Design review of the part built by this model. Coordinates are the model's own, in mm. A direction names the side the tool comes from. Coordinates: 2 decimals unless noted, no trailing zeros. Write each loop counter-clockwise with the first axis right and the second up, starting at its lowest first coordinate (ties: lowest second). Pieces come first, ordered by that corner, then holes. Notation, with made-up numbers: (22, 67.25) -> (34, 67.25) arc R23 ccw to (34, 82.25) -> close; hole circle Ø11 at (24, -15). An arc over 180 degrees is marked (long way). One line per question, with ' | ' between items. Start each with the question number.
Q1. Wall thickness on probe 1 along Z at (x, y) = (57.15, 2.25); probe 2 along X at (y, z) = (4.5, -6.55) (3 decimals); probe 3 along X at (y, z) = (5, 25.4) (3 decimals): over which ranges is each line inside the solid? List them lowest first.
Q2. For faces 1 (the flat face through (27, 3, 0)), 2 (the cylindrical face through (55.563, 3.131, 26.617)), list the 3-axis set-ups (+Z, -Z, +X, -X, +Y, -Y) from which the entire face can be reached by the end or side of a thin tool; tool diameter is ignored.
Q3. Add section C-C on z = -19.05. State the section outline as (x, y) points (3 decimals), and give its area (3 significant figures).
Q4. Add section D-D on y = 3. State the section outline as (x, z) points (3 decimals).
Q5. For P1, Ø1.9, axis at x = 37, y = 3, coming from the +Z side, flat-tipped, find the tip position at first contact; note if it passes through.
Q6. Add section A-A on z = -6.55. State the section outline as (x, y) points (3 decimals), and give its area (3 significant figures).
Q7. Add section B-B on x = 57.15. State the section outline as (y, z) points.
from build123d import *

# Parameters (mm, degrees)
SKETCH1_R           = 2
BOSS_EXTRUDE1_DEPTH = 6.35


with BuildPart() as part:
    # Sketch1 → Boss-Extrude1 (new body)
    with BuildSketch(Plane(origin=(0, 0, 0), x_dir=(1, 0, 0), z_dir=(0, 1, 0))):
        Polygon((0, 38.1), (0, 0), (53.975, 0), (53.975, -82.55), (88.9, -82.55), (88.9, 0), (88.9, 38.1), (53.975, 38.1), align=None)
        with Locations((57.15, -76.2)):
            Circle(SKETCH1_R, mode=Mode.SUBTRACT)
        with Locations((57.15, -25.4)):
            Circle(SKETCH1_R, mode=Mode.SUBTRACT)
        with Locations((16.075, 6.55)):
            Circle(SKETCH1_R, mode=Mode.SUBTRACT)
        with Locations((41.075, 6.55)):
            Circle(SKETCH1_R, mode=Mode.SUBTRACT)
        with Locations((16.075, 31.55)):
            Circle(SKETCH1_R, mode=Mode.SUBTRACT)
        with Locations((28.575, 19.05)):
            Circle(SKETCH1_R, mode=Mode.SUBTRACT)
        with Locations((41.075, 31.55)):
            Circle(SKETCH1_R, mode=Mode.SUBTRACT)
    extrude(amount=BOSS_EXTRUDE1_DEPTH)


solid = part.part
Output values:
1) probe 1: z = -38.1 to 23.4, 27.4 to 74.2, 78.2 to 82.55 | probe 2: x = 0 to 14.075, 18.075 to 39.075, 43.075 to 88.9 | probe 3: x = 53.975 to 55.15, 59.15 to 88.9
2) face 1: +Z, -X, +Y, -Y | face 2: +Y, -Y
3) outline: (0, 0) -> (26.575, 0) -> (26.575, 6.35) -> (0, 6.35) -> close; (30.575, 0) -> (88.9, 0) -> (88.9, 6.35) -> (30.575, 6.35) -> close | area: 539 mm2
4) outline: (0, -38.1) -> (88.9, -38.1) -> (88.9, 82.55) -> (53.975, 82.55) -> (53.975, 0) -> (0, 0) -> close; hole circle Ø4 at (16.075, -31.55); hole circle Ø4 at (16.075, -6.55); hole circle Ø4 at (28.575, -19.05); hole circle Ø4 at (41.075, -31.55); hole circle Ø4 at (41.075, -6.55); hole circle Ø4 at (57.15, 25.4); hole circle Ø4 at (57.15, 76.2)
5) P1: stops at z = 0
6) outline: (0, 0) -> (14.075, 0) -> (14.075, 6.35) -> (0, 6.35) -> close; (18.075, 0) -> (39.075, 0) -> (39.075, 6.35) -> (18.075, 6.35) -> close; (43.075, 0) -> (88.9, 0) -> (88.9, 6.35) -> (43.075, 6.35) -> close | area: 514 mm2
7) outline: (0, -38.1) -> (6.35, -38.1) -> (6.35, 23.4) -> (0, 23.4) -> close; (0, 27.4) -> (6.35, 27.4) -> (6.35, 74.2) -> (0, 74.2) -> close; (0, 78.2) -> (6.35, 78.2) -> (6.35, 82.55) -> (0, 82.55) -> close
